Could you check a few things on this model? Use its own coordinates, in mm. A direction names the side the tool comes from. Coordinates: 2 decimals unless noted, no trailing zeros. Loops run counter-clockwise (first coordinate to the right, second up) from the corner with the lowest first, then second, coordinate; pieces in that order, holes last. Notation, with made-up numbers: (2, 66) - (60, 66) arc R9 cw to (60, 70) - close; hole circle Ø6 at (68.25, -5). An arc over 180 degrees is marked (long way). One line per item, written item: value. Start each with the question number.
(1) If we section it at B-B on x = 8.75: Write out the boundary of the cut face in (y, z), then the cut area to 3 significant figures.
(2) If we section it at A-A on z = 9: Write out the boundary of the cut face in (x, y).
(3) If we section it at C-C on x = 15.25: Count the separate pieces of the cut face and the enclosed holes in it, then the cut area to 3 significant figures.
(4) On a 3-axis mill with a long thin cutter (end or side, diameter ignored), from which of +Z, -Z, +X, -X, +Y, -Y can I reach the whole of each face in a straight line? I mean faces 4 (the face through (11, 44, 6.883)), 5 (the face through (14.79, 6.453, 9.93)), 6 (the face through (14.79, -33.276, 10.337)). Say none if no direction works.
(5) If we section it at D-D on y = 28.5: Write out the boundary of the cut face in (x, z).
(6) I'm going to push flat-ended pins straight in: P1, Ø3, axis at x = 18.5, y = 28.5, coming from the +Z side; P2, Ø6, axis at x = 7.5, y = -43.5, coming from the +Z side; P3, Ø1, axis at y = -30.5, z = 12.5, coming from the -X side; P4, Ø3, axis at x = 21, y = -61, coming from the +Z side. Where does each tip first touch, or does it pass through?
(7) If I drill on line 1 along Y through (x, z) = (16, 9.75); line 2 along Y through (x, z) = (1.75, 7.5); line 3 along Z through (x, y) = (16.5, -101.5), over which ranges is the centre line in solid material (lowest first)? Write a range as from..to.
(8) If we mould it in two halves opening along X, with no side actions, what happens to faces 1 (the face through (14.79, -53.74, 9.52)), 2 (the face through (30, -35, 5)), 3 (the face through (15.878, -110.723, 3.35))? For each: pulls with the +X half, pulls with the -X half, needs draft (parallel to the pull), parting line crosses it, or undercut.
```python
from build123d import *

# Parameters (mm, degrees)
F1_DEPTH       = 30
F2_R           = 2
F3_R           = 1
F5_D           = 5
F5_CSINK_D     = 8
F5_CSINK_ANGLE = 90
F7_D           = 5
F7_CSINK_D     = 8
F7_CSINK_ANGLE = 90


with BuildPart() as f1:
    # F0 (on Right) → F1 (new body)
    with BuildSketch(Plane.YZ):
        with BuildLine():
            Line((-114.335611, 1.639002), (-103.282312, 1.639002))
            Line((-103.282312, 1.639002), (-103.19238, 1.639002))
            Line((-103.19238, 1.639002), (36.717688, 1.639002))
            Line((36.717688, 1.639002), (46.717688, 1.639002))
            Line((46.717688, 1.639002), (46.717688, 5.639002))
            Line((46.717688, 5.639002), (46.717688, 6.883289))
            Line((46.717688, 6.883289), (36.389513, 6.883289))
            ThreePointArc((36.389513, 6.883289), (36.026758, 11.097664), (36.776017, 15.260735))
            Line((36.776017, 15.260735), (16.717688, 6.883289))
            Line((16.717688, 6.883289), (6.915737, 6.856559))
            ThreePointArc((6.915737, 6.856559), (6.430977, 10.892172), (6.974065, 14.92035))
            Line((6.974065, 14.92035), (-12.459779, 6.803723))
            Line((-12.459779, 6.803723), (-23.238242, 6.77433))
            ThreePointArc((-23.238242, 6.77433), (-23.658847, 10.684605), (-23.117268, 14.579968))
            Line((-23.117268, 14.579968), (-41.928537, 6.723361))
            Line((-41.928537, 6.723361), (-53.387725, 6.692112))
            ThreePointArc((-53.387725, 6.692112), (-53.747579, 10.476515), (-53.208595, 14.239585))
            Line((-53.208595, 14.239585), (-71.397287, 6.643))
            Line((-71.397287, 6.643), (-83.343368, 6.610423))
            ThreePointArc((-83.343368, 6.610423), (-83.671143, 10.325154), (-83.134051, 14.015437))
            Line((-83.134051, 14.015437), (-100.864061, 6.610423))
            Line((-100.864061, 6.610423), (-114.335611, 6.610423))
            Line((-114.335611, 6.610423), (-114.335611, 1.639002))
        make_face()
    extrude(amount=F1_DEPTH)

    # F2
    f2_edges = [f1.edges().sort_by_distance(p)[0] for p in [
        (0, -114.335611, 4.124713),
        (30, -114.335611, 4.124713),
        (0, 46.717688, 4.261146),
        (30, 46.717688, 4.261146),
    ]]
    fillet(f2_edges, radius=F2_R)

    # F3
    f3_edges = [f1.edges().sort_by_distance(p)[0] for p in [
        (15, 36.776017, 15.260735),
        (15, 6.974065, 14.92035),
        (15, -23.117268, 14.579968),
        (15, -53.208595, 14.239585),
        (15, -83.134051, 14.015437),
    ]]
    fillet(f3_edges, radius=F3_R)

    # F5 (through all)
    with Locations(Plane.XY.offset(6.610423)):
        with Locations((15.335711, -108.282417)):
            CounterSinkHole(F5_D / 2, F5_CSINK_D / 2, counter_sink_angle=F5_CSINK_ANGLE)

    # F7 (through all)
    with Locations(Plane.XY.offset(6.883289)):
        with Locations((15.114769, 41.508552)):
            CounterSinkHole(F7_D / 2, F7_CSINK_D / 2, counter_sink_angle=F7_CSINK_ANGLE)


solid = f1.part
```
Values:
1. outline: (-114.34, 1.64) - (46.72, 1.64) - (46.72, 6.88) - (36.39, 6.88) arc R16.07 cw to (36.3, 13.38) arc R1 ccw to (34.93, 14.49) - (16.72, 6.88) - (6.92, 6.86) arc R16.07 cw to (6.6, 13.12) arc R1 ccw to (5.23, 14.19) - (-12.46, 6.8) - (-23.24, 6.77) arc R16.07 cw to (-23.49, 12.78) arc R1 ccw to (-24.86, 13.85) - (-41.93, 6.72) - (-53.39, 6.69) arc R16.07 cw to (-53.58, 12.44) arc R1 ccw to (-54.95, 13.51) - (-71.4, 6.64) - (-83.34, 6.61) arc R16.07 cw to (-83.51, 12.22) arc R1 ccw to (-84.88, 13.29) - (-100.86, 6.61) - (-114.34, 6.61) - close
1. area: 1,170 mm2
2. outline: (0, -95.14) - (30, -95.14) - (30, -83.65) - (0, -83.65) - close; (0, -65.75) - (30, -65.75) - (30, -53.71) - (0, -53.71) - close; (0, -36.48) - (30, -36.48) - (30, -23.6) - (0, -23.6) - close; (0, -7.2) - (30, -7.2) - (30, 6.53) - (0, 6.53) - close; (0, 21.79) - (30, 21.79) - (30, 36.07) - (0, 36.07) - close
3. separate pieces: 3
3. enclosed holes: 0
3. area: 1,120 mm2
4. face 4: +Z, +X, -X, +Y
4. face 5: +X, -X
4. face 6: +Z, +X, -X
5. outline: (0, 1.64) - (30, 1.64) - (30, 11.8) - (0, 11.8) - close
6. P1: stops at z = 12.43
6. P2: stops at z = 7.32
6. P3: passes through
6. P4: stops at z = 11.61
7. line 1: y = -93.35..-83.68, -63.96..-53.75, -34.68..-23.65, -5.41..6.46, 23.58..36.02
7. line 2: y = -98.73..-83.5, -69.35..-53.54, -40.07..-23.39, -10.79..6.77, 18.19..36.27
7. line 3: z = 1.64..6.61
8. face 1: needs draft
8. face 2: pulls with the +X half
8. face 3: undercut
